```python
from build123d import *

# Parameters (mm, degrees)
BOSS_EXTRUDE1_DEPTH = 9.525
SKETCH3_W           = 9.525
SKETCH3_H           = 12.7
CUT_EXTRUDE1_DEPTH  = 9.525
SKETCH4_W           = 9.525
SKETCH4_H           = 12.7
CUT_EXTRUDE2_DEPTH  = 9.525
SKETCH5_W           = 9.525
SKETCH5_H           = 12.7
CUT_EXTRUDE3_DEPTH  = 9.525


with BuildPart() as part:
    # Sketch2 → Boss-Extrude1 (new body)
    with BuildSketch(Plane(origin=(0, 0, 0), x_dir=(0, 0, -1), z_dir=(1, 0, 0))):
        Polygon((-73.252839905, 0), (-64.170161704, 37.001553436), (-37.001553436, 63.712538532), (0, 72.795216732), (37.001553436, 63.712538532), (64.170161704, 37.001553436), (73.252839905, 0), align=None)
    extrude(amount=BOSS_EXTRUDE1_DEPTH)

    # Sketch3 → Cut-Extrude1 (cut)
    with BuildSketch(Plane(origin=(0, 16.959318632, 69.089878642), x_dir=(1, 0, 0), z_dir=(0, 0.238390504, 0.971169382))):
        with Locations((4.7625, 1.58721858)):
            Rectangle(SKETCH3_W, SKETCH3_H)
    cut_extrude1 = extrude(amount=-CUT_EXTRUDE1_DEPTH, mode=Mode.SUBTRACT)

    # Sketch4 → Cut-Extrude2 (cut)
    with BuildSketch(Plane(origin=(0, 50.895476621, 50.038202327), x_dir=(1, 0, 0), z_dir=(0, 0.713086831, 0.701075724))):
        with Locations((4.7625, -0.768006391)):
            Rectangle(SKETCH4_W, SKETCH4_H)
    cut_extrude2 = extrude(amount=-CUT_EXTRUDE2_DEPTH, mode=Mode.SUBTRACT)

    # Sketch5 → Cut-Extrude3 (cut)
    with BuildSketch(Plane(origin=(0, 68.658262209, 16.853370832), x_dir=(1, 0, 0), z_dir=(0, 0.971169382, 0.238390504))):
        with Locations((4.7625, -1.696311598)):
            Rectangle(SKETCH5_W, SKETCH5_H)
    cut_extrude3 = extrude(amount=-CUT_EXTRUDE3_DEPTH, mode=Mode.SUBTRACT)

    # Mirror1: Cut-Extrude1, Cut-Extrude2, Cut-Extrude3 across plane
    add(cut_extrude1.mirror(Plane.XY), mode=Mode.SUBTRACT)
    add(cut_extrude2.mirror(Plane.XY), mode=Mode.SUBTRACT)
    add(cut_extrude3.mirror(Plane.XY), mode=Mode.SUBTRACT)


solid = part.part
```
Geometry: final body of the model. Coordinates: model frame, mm. A direction names the side the tool comes from. Round coordinates to 2 decimals unless told otherwise and drop trailing zeros. Order: outer loops, then holes, each group sorted by start corner. A loop starts at its lowest first (then second) coordinate and runs counter-clockwise, first axis right, second up. Notation, with made-up numbers: (13, 44) - (54, 44) arc R13 cw to (54, 67) - close; hole circle Ø1 at (25, -7). An arc over 180 degrees is marked (long way). Write item = value, one per line. Start each with the question number.
Q1. Access query for faces 1 (the flat face through (4.696, 11.214, 65.665)), 2 (the flat face through (4.7, 62.18, -23.55)), 3 (the flat face through (4.696, 51.46, 42.766)). Directions: +Z, -Z, +X, -X, +Y, -Y. A direction counts if a zero-diameter tool reaches every point of the face in a straight line with its end or side. Return the directions, or none.
Q2. Pin query (flat end, axial travel): pin 1 (5 mm diameter, centred on x = 7.5, z = -13, fed in from +Y); pin 2 (1 mm diameter, centred on x = 6.5, z = -24.5, fed in from +Y); pin 3 (4 mm diameter, centred on x = 2, y = 53.5, fed in from +Z). Return the tip coordinate at first contact, or that it passes through.
Q3. Ray query, line 1 (Y direction, x = 6, z = -40); line 2 (Z direction, x = 2, y = 41); line 3 (Z direction, x = 4.25, y = 37). Return the intervals inside material, ascending. Write a range as from..to.
Q4. Pull-direction query (Y, two-part tool) for faces 4 (the flat face through (5, 0, -1)), 5 (the flat face through (4.7, 59.32, -41.47)), 6 (the flat face through (4.696, 51.46, -42.766)); classes: +Y half, -Y half, draft (parallel to the pull), parting line (faces both ways), or undercut.
Q5. Cut plane C-C on y = 26.5. Return the cut outline in (x, z) (3 decimals), and give its area (3 significant figures).
Q6. Cut plane B-B on z = 31.5. Return the cut outline in (x, y) (3 decimals), and give its area (3 significant figures).
Outcome:
q1.face_1 = +X, -X
q1.face_2 = +X, -X, +Y
q1.face_3 = +Z, +X, -X
q2.pin_1 = 70.22
q2.pin_2 = 66.74
q2.pin_3 = 46.06
q3.line_1 = 0..47.41, 48.65..60.76
q3.line_2 = -60.1..-50.29, -46.52..46.52, 50.29..60.1
q3.line_3 = -64.17..64.17
q4.face_4 = -Y half
q4.face_5 = +Y half
q4.face_6 = undercut
q5.outline = (0, -66.748) - (9.525, -66.748) - (9.525, 66.748) - (0, 66.748) - close
q5.area = 1,270 mm^2
q6.outline = (0, 0) - (9.525, 0) - (9.525, 65.063) - (0, 65.063) - close
q6.area = 620 mm^2
